Geometry check sheet. Reference: the model listing, model coordinates, mm. A direction names the side the tool comes from. Give positions to 0.01 mm unless a question says otherwise; leave off trailing zeros. Order: outer loops, then holes, each group sorted by start corner. A loop starts at its lowest first (then second) coordinate and runs counter-clockwise, first axis right, second up.
from build123d import *

# Parameters (mm, degrees)
SKETCH1_W           = 15
SKETCH1_H           = 17
BOSS_EXTRUDE1_DEPTH = 36
SKETCH2_W           = 11
SKETCH2_H           = 36
CUT_EXTRUDE1_DEPTH  = 15
SKETCH3_W           = 15
SKETCH3_H           = 30
CUT_EXTRUDE2_DEPTH  = 15


with BuildPart() as part:
    # Sketch1 → Boss-Extrude1 (new body)
    with BuildSketch(Plane.XY):
        Rectangle(SKETCH1_W, SKETCH1_H)
    extrude(amount=BOSS_EXTRUDE1_DEPTH)

    # Sketch2 → Cut-Extrude1 (cut)
    with BuildSketch(Plane(origin=(0, 8.5, 0), x_dir=(1, 0, 0), z_dir=(0, 1, 0))):
        with Locations((0, -18)):
            Rectangle(SKETCH2_W, SKETCH2_H)
    extrude(amount=-CUT_EXTRUDE1_DEPTH, mode=Mode.SUBTRACT)

    # Sketch3 → Cut-Extrude2 (cut)
    with BuildSketch(Plane(origin=(0, 8.5, 0), x_dir=(1, 0, 0), z_dir=(0, 1, 0))):
        with Locations((0, -18)):
            Rectangle(SKETCH3_W, SKETCH3_H)
    extrude(amount=-CUT_EXTRUDE2_DEPTH, mode=Mode.SUBTRACT)


solid = part.part
Item 1: Draft check along Z on faces 1 (the flat face through (0, -7, 36)), 2 (the flat face through (-7, 8.5, 34)), 3 (the flat face through (-7, 1, 33)). Enter one of: released by +Z, released by -Z, zero draft, split by the parting line, or undercut.
Reported:
face 1: released by +Z
face 2: zero draft
face 3: undercut
Item 2: Scan lines: L1, parallel to Z at x = 6, y = 4.5; L2, parallel to Y at x = -4, z = 22.5. Record each from-to range of solid material in increasing order.
Reported:
L1: z = 0 to 3, 33 to 36
L2: y = -8.5 to -6.5
Item 3: Sectioned sample at C-C (z = 31). Enter the section's corners in (x, y).
Reported:
outline: (-7.5, -8.5) - (7.5, -8.5) - (7.5, -6.5) - (-7.5, -6.5) - close
Item 4: Set-up check for faces 4 (the flat face through (-5.5, 1, 2)), 5 (the flat face through (-7, 1, 3)), 6 (the flat face through (7.5, -7, 18)): record each of +Z, -Z, +X, -X, +Y, -Y from which the full face is reachable in a straight line by a thin tool's end or side.
Reported:
face 4: +Z, -Z, +Y
face 5: +X, -X, +Y
face 6: +Z, -Z, +X, +Y, -Y
Item 5: Sectioned sample at A-A (y = -1). Enter the section's corners in (x, z).
Reported:
outline: (-7.5, 0) - (-5.5, 0) - (-5.5, 3) - (-7.5, 3) - close; (-7.5, 33) - (-5.5, 33) - (-5.5, 36) - (-7.5, 36) - close; (5.5, 0) - (7.5, 0) - (7.5, 3) - (5.5, 3) - close; (5.5, 33) - (7.5, 33) - (7.5, 36) - (5.5, 36) - close
Item 6: Sectioned sample at B-B (x = -6). Enter the section's corners in (y, z), and give its area (3 significant figures).
Reported:
outline: (-8.5, 0) - (8.5, 0) - (8.5, 3) - (-6.5, 3) - (-6.5, 33) - (8.5, 33) - (8.5, 36) - (-8.5, 36) - close
area: 162 mm2
Item 7: Gauge pin test, flat end, axial feed: pin 1 (3 mm diameter, centred on x = -0.5, z = 21, fed in from +Y). Record the tip position at first contact, or that the pin passes through.
Reported:
pin 1: stops at y = -6.5
Item 8: Sectioned sample at D-D (x = 0.5). Enter the section's corners in (y, z), and give its area (3 significant figures).
Reported:
outline: (-8.5, 0) - (-6.5, 0) - (-6.5, 36) - (-8.5, 36) - close
area: 72.0 mm2
